Model file for the job. Use its own axes, mm. Round coordinates to 2 decimals unless told otherwise and drop trailing zeros. Loops run counter-clockwise (first coordinate to the right, second up) from the corner with the lowest first, then second, coordinate; pieces in that order, holes last. Notation, with made-up numbers: (52, 82.5) - (87, 82.5) arc R10 ccw to (87, 98.5) - close; hole circle Ø1 at (0.5, -15.75). An arc over 180 degrees is marked (long way). Answer as a JSON object with one key per item and string values.
from build123d import *

# Parameters (mm, degrees)
SKETCH_2_W      = 98
SKETCH_2_H      = 98
EXTRUDE_1_DEPTH = 10
SKETCH_3_W      = 98
SKETCH_3_H      = 125
EXTRUDE_2_DEPTH = 10
SKETCH_4_W      = 98
SKETCH_4_H      = 62.5
EXTRUDE_3_DEPTH = 886.75
SKETCH_5_W      = 98
SKETCH_5_H      = 62.5
EXTRUDE_4_DEPTH = 7.1
SKETCH_6_W      = 98
SKETCH_6_H      = 62.5
EXTRUDE_5_DEPTH = 7.1
SKETCH_9_W      = 115.1
SKETCH_9_H      = 3.2
EXTRUDE_6_DEPTH = 102


with BuildPart() as part:
    # 草图2 → 凸台-拉伸1 (new body)
    with BuildSketch(Plane(origin=(0, 0, 0), x_dir=(1, 0, 0), z_dir=(0, 1, 0))):
        with Locations((34.507061985, 30.744472309)):
            Rectangle(SKETCH_2_W, SKETCH_2_H)
    extrude(amount=EXTRUDE_1_DEPTH)

    # 草图3 → 凸台-拉伸2 (add)
    with BuildSketch(Plane.XY.offset(18.255527691)):
        with Locations((34.507061985, -52.5)):
            Rectangle(SKETCH_3_W, SKETCH_3_H)
    extrude(amount=EXTRUDE_2_DEPTH)

    # 草图4 → 凸台-拉伸3 (add)
    with BuildSketch(Plane.XY.offset(28.255527691)):
        with Locations((34.507061985, -83.75)):
            Rectangle(SKETCH_4_W, SKETCH_4_H)
    extrude(amount=EXTRUDE_3_DEPTH)

    # 镜向4: part across plane


with BuildPart() as part_1:
    add(part.part)
    add(part.part.mirror(Plane.XY.offset(915.005527691)))

    # 草图5 → 凸台-拉伸4 (add)
    with BuildSketch(Plane.XY.offset(28.255527691)):
        with Locations((34.507061985, -21.25)):
            Rectangle(SKETCH_5_W, SKETCH_5_H)
    extrude(amount=EXTRUDE_4_DEPTH)

    # 草图6 → 凸台-拉伸5 (add)
    with BuildSketch(Plane(origin=(0, 0, 1801.755527691), x_dir=(-1, 0, 0), z_dir=(0, 0, -1))):
        with Locations((-34.507061985, -21.25)):
            Rectangle(SKETCH_6_W, SKETCH_6_H)
    extrude(amount=EXTRUDE_5_DEPTH)

    # 草图9 → 凸台-拉伸6 (add)
    with BuildSketch(Plane.ZY.offset(14.492938015)):
        with Locations((-22.194472309, 8.4)):
            Rectangle(SKETCH_9_W, SKETCH_9_H)
        with Locations((1852.205527691, 8.4)):
            Rectangle(SKETCH_9_W, SKETCH_9_H)
    extrude(amount=EXTRUDE_6_DEPTH)


solid = part_1.part
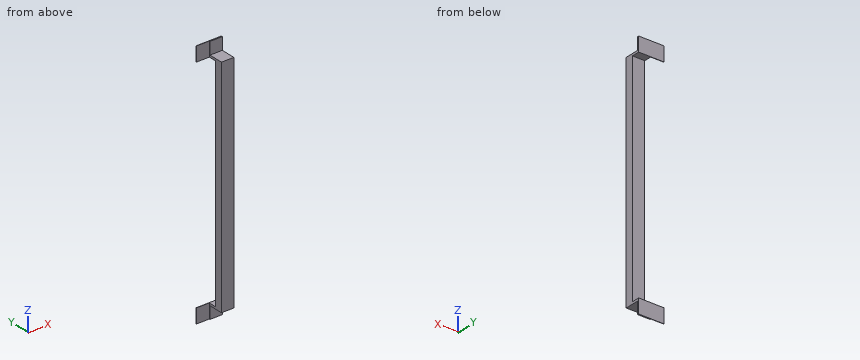
1) Drop flat-ended pins along their axis: P1, Ø1, axis at x = 22, z = 991, coming from the +Y side; P2, Ø19, axis at x = 18, y = -36, coming from the +Z side; P3, Ø8, axis at y = -95.5, z = 648.5, coming from the -X side. Give the stop position or say it passes through.
Values follow:
{"P1": "y = -52.5", "P2": "z = 1811.76", "P3": "x = -14.49"}
2) Slice it at D-D on z = 1452.5. List the corners of the cut face in (x, y), then the cut area to 4 significant figures.
Values follow:
{"outline": "(-14.49, -115) - (83.51, -115) - (83.51, -52.5) - (-14.49, -52.5) - close", "area": "6,125 mm²"}
3) Slice it at B-B on y = -20.5. List the corners of the cut face in (x, z), then the cut area to 3 significant figures.
Values follow:
{"outline": "(-14.49, 18.26) - (83.51, 18.26) - (83.51, 35.36) - (-14.49, 35.36) - close; (-14.49, 1794.66) - (83.51, 1794.66) - (83.51, 1811.76) - (-14.49, 1811.76) - close", "area": "3,350 mm²"}
4) Slice it at C-C on x = 40. List the corners of the cut face in (y, z).
Values follow:
{"outline": "(-115, 18.26) - (0, 18.26) - (0, -79.74) - (10, -79.74) - (10, 35.36) - (-52.5, 35.36) - (-52.5, 1794.66) - (10, 1794.66) - (10, 1909.76) - (0, 1909.76) - (0, 1811.76) - (-115, 1811.76) - close"}
5) Probe probe 1 along Z at (x, y) = (33.5, -40); probe 2 along X at (y, z) = (-56, 773); probe 3 along Y at (x, z) = (25.5, 1466). List the from-to ranges inside material, lowest first.
Values follow:
{"probe 1": "18.26 to 35.36, 1794.66 to 1811.76", "probe 2": "-14.49 to 83.51", "probe 3": "-115 to -52.5"}
6) Slice it at A-A on x = -89. List the corners of the cut face in (y, z).
Values follow:
{"outline": "(6.8, -79.74) - (10, -79.74) - (10, 35.36) - (6.8, 35.36) - close; (6.8, 1794.66) - (10, 1794.66) - (10, 1909.76) - (6.8, 1909.76) - close"}
